Autodesk Inventor part; units mm, degrees
ref_plane "Work Plane1" through (0, 15, 0) normal (0, 1, 0) x (-1, 0, 0)
ref_plane "YZ Plane" through (0, 0, 0) normal (1, 0, 0) x (0, 1, 0)
ref_plane "XY Plane" through (0, 0, 0) normal (0, 0, 1) x (1, 0, 0)
sketch "Sketch1" plane through (0, 0, 0) normal (0, 1, 0) x (-1, 0, 0)
  line L0 (32.75, 5) -> (33.95, 5)
  line L1 (33.95, 5) -> (33.95, 85)
  line L2 (33.95, 85) -> (34.25, 85)
  line L3 (34.25, 85) -> (34.25, 135)
  line L4 (34.25, 135) -> (34.75, 135)
  line L5 (34.75, 135) -> (34.75, 205)
  line L6 (34.75, 205) -> (33.75, 205)
  line L7 (33.75, 205) -> (33.75, 245)
  line L8 (33.75, 245) -> (33.75, 245)
  line L9 (33.75, 245) -> (33.75, 350)
  line L10 (33.75, 350) -> (0, 350)
  line L11 (0, 189.8856) -> (0, -122.7414) construction
  line L12 (32.75, 5) -> (32.75, 0)
  line L13 (0, 350) -> (0, 0)
  line L14 (32.75, 0) -> (32.95, 0)
  line L15 (32.95, 0) -> (32.95, -4)
  line L16 (32.95, -4) -> (34.65, -4)
  line L17 (34.65, -4) -> (34.65, -54)
  line L18 (34.65, -54) -> (34.85, -54)
  line L19 (34.85, -54) -> (34.85, -134)
  line L20 (34.85, -134) -> (0, -134)
  line L21 (0, 0) -> (0, -134)
  line L22 (32.75, 0) -> (32.95, 0)
  dimension "d0" = 105
  dimension "d3" = 70
  dimension "d2" = 80
  dimension "d4" = 5
  dimension "d15" = 40
  dimension "d16" = 50
  dimension "d69" = 33.75
  dimension "d70" = 34.75
  dimension "d71" = 33.95
  dimension "d78" = 32.75
  dimension "d82" = 4
  dimension "d83" = 50
  dimension "d84" = 32.95
  dimension "d85" = 34.85
  dimension "d86" = 80
  dimension "d87" = 33.75
  dimension "d88" = 34.25
  dimension "d89" = 34.65
ref_plane "Work Plane1" through (0, 15, 0) normal (0, 1, 0) x (-1, 0, 0)
sketch "Sketch2" plane through (0, 15, 0) normal (0, 1, 0) x (-1, 0, 0)
  arc A0 (-5, 259) -> (5, 259) centre (0, 259) ccw
  arc A1 (5, 334) -> (-5, 334) centre (0, 334) ccw
  line L0 (-5, 334) -> (-5, 259)
  line L1 (5, 334) -> (5, 259)
  line L2 (0, 0) -> (0, 401.4271) construction
  dimension "d18" = 10
  dimension "d19" = 10
  dimension "d65" = 259
  dimension "d68" = 75
sketch "Sketch3" plane through (0, 15, 0) normal (0, 1, 0) x (-1, 0, 0)
  circle A0 centre (0, -79) radius 7
  point P0 (0, 0)
  dimension "d22" = 14
  dimension "d66" = 79
sketch "Sketch4" plane through (0, 0, 0) normal (1, 0, 0) x (0, 1, 0)
  circle A0 centre (0, -114) radius 7
  point P0 (0, 0)
  dimension "d28" = 14
  dimension "d67" = 114
revolve "Revolution1" add sketch "Sketch1" angle 360 about axis through (0, 0, 350) along (0, 0, -1)
extrude "Extrusion4" cut sketch "Sketch2" along normal blind 10
extrude "Extrusion5" cut sketch "Sketch3" along normal blind 20 and the other way blind 45
extrude "Extrusion6" cut sketch "Sketch4" along normal blind 35 and the other way blind 30
sketch "Sketch5" plane through (0, 0, 0) normal (0, 1, 0) x (-1, 0, 0)
  line L0 (32.75, 5) -> (32.75, 0)
  point P0 (0, 0)
sketch "Sketch6" plane through (0, 0, 0) normal (1, 0, 0) x (0, 1, 0)
  line L0 (0, 0) -> (-46.2751, 0) construction
equation "\"espesor_testero\" = 4"
equation "\"espesor_brida\" = 5"
properties part number "Mangon_Conduccion"
Can you work these out from the model? Positions are in its coordinate system, mm. A direction names the side the tool comes from. Give positions to 0.01 mm unless a question says otherwise; leave off trailing zeros. Order: outer loops, then holes, each group sorted by start corner. A loop starts at its lowest first (then second) coordinate and runs counter-clockwise, first axis right, second up. Notation, with made-up numbers: M 3.25,63 L 13.25,63 A23 ccw 13.25,99 Z; hole C 80,-35.5 d9. An arc over 180 degrees is marked long. Use a Markdown table: item, result. Add a question column.
Item 1: Suppose I cut it at C-C (z = 181). List the corners of the cut face in (x, y) for me, then the cut area to 3 significant figures.
Item 2: Will these pins go through, and if not, where does the flat tip stop? pin 1 (11 mm diameter, centred on y = 0.5, z = -113, fed in from +X); pin 2 (2 mm diameter, centred on x = 7.5, z = 167.5, fed in from +Y); pin 3 (4 mm diameter, centred on x = 0.5, z = -76, fed in from +Y).
Item 3: For faces 1 (the cylindrical face through (26.78, 20.54, 278.52)), 2 (the flat face through (0, 0, 350)), 3 (the flat face through (-31, -13, -4)), which set-ups out of +Z, -Z, +X, -X, +Y, -Y let a thin tool reach every point of the face, with its end or its side?
Item 4: If I drill on L1, parallel to Z at x = 0, y = 19; L2, parallel to Y at x = 2.5, z = -114; L3, parallel to Z at x = 18, y = -28, over which ranges is the centre line in solid material (lowest first)? Write a range as [from, to].
Item 5: Suppose I cut it at D-D (z = -58). List the corners of the cut face in (x, y) for me, then the cut area to 3 significant figures.
Item 6: We'd pull the mould along Z, two halves only. Please class faces 4 (the cylindrical face through (0.91, 1.97, -85.94)), 5 (the flat face through (0, 0, -134)): +Z half, -Z half, draft (parallel to the pull), parting line (faces both ways), or undercut.
Answer sheet:
| question | item | result |
|---|---|---|
| 1 | outline | C 0,0 d69.5 |
| 1 | area | 3,790 mm² |
| 2 | pin 1 | stops at x = -30 |
| 2 | pin 2 | stops at y = 34.14 |
| 2 | pin 3 | stops at y = -30 |
| 3 | face 1 | +Z |
| 3 | face 2 | +Z, +X, -X, +Y, -Y |
| 3 | face 3 | none |
| 4 | L1 | z = [-134, -86], [-72, 254], [339, 350] |
| 4 | L2 | y = [-34.76, -7], [7, 34.76] |
| 4 | L3 | z = [-134, -4], [5, 350] |
| 5 | outline | C 0,0 d69.7 |
| 5 | area | 3,820 mm² |
| 6 | face 4 | undercut |
| 6 | face 5 | -Z half |
